Verification items for the finished model (mm, model axes). Coordinates: 2 decimals unless noted, no trailing zeros. Order: outer loops, then holes, each group sorted by start corner. A loop starts at its lowest first (then second) coordinate and runs counter-clockwise, first axis right, second up. Notation, with made-up numbers: M 9,-39 L 50,-39 A24 cw 50,-2 Z; hole C 80.5,7.25 d11. An arc over 180 degrees is marked long. Answer as a JSON object with one key per item and string values. Group by question number.
(1) Cross-section at C-C (y = -2.3). Enter the section's corners in (x, z).
(2) Cross-section at B-B (z = -12). Enter the section's corners in (x, y), plus the area to 3 significant figures.
(3) Cross-section at D-D (x = -10). Enter the section's corners in (y, z), plus the area to 3 significant figures.
(4) Cross-section at A-A (x = 0). Enter the section's corners in (y, z), plus the area to 3 significant figures.
(5) Material ranges on line 1 (Z direction, x = 0, y = 0.95); line 2 (X direction, y = -2.65, z = -1); line 3 (Y direction, x = 2, z = 2.5), recorded low to high.
(6) Gauge pin test, flat ends, axial feed: pin 1 Ø1.5 at (x, y) = (-21.5, -1) entering from +Z; pin 2 Ø2 at (x, y) = (-0.5, -2.5) entering from -Z; pin 3 Ø2.5 at (y, z) = (-2.5, -0.5) entering from -X; pin 4 Ø1.5 at (y, z) = (-1, 0) entering from +X. Record the tip position at first contact, or that the pin passes through.
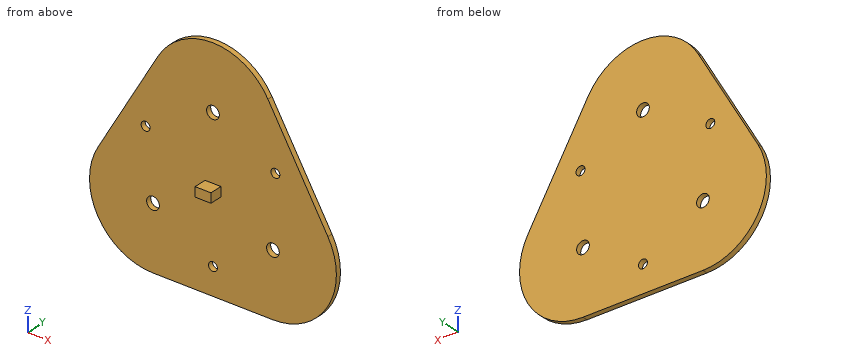
from build123d import *

# Parameters (mm, degrees)
SKETCH1_R           = 2
SKETCH1_R_2         = 1.4
BOSS_EXTRUDE1_DEPTH = 1.65
SKETCH2_W           = 5
SKETCH2_H           = 3
BOSS_EXTRUDE2_DEPTH = 4


with BuildPart() as part:
    # Sketch1 → Boss-Extrude1 (new body)
    with BuildSketch(Plane(origin=(0, 0, 0), x_dir=(1, 0, 0), z_dir=(0, 1, 0))):
        with BuildLine():
            Line((36.224008076, 0.913940814), (17.320508076, -31.827881627))
            ThreePointArc((17.320508076, -31.827881627), (0, -41.827881627), (-17.320508076, -31.827881627))
            Line((-17.320508076, -31.827881627), (-36.224008076, 0.913940814))
            ThreePointArc((-36.224008076, 0.913940814), (-36.224008076, 20.913940814), (-18.9035, 30.913940814))
            Line((-18.9035, 30.913940814), (18.9035, 30.913940814))
            ThreePointArc((18.9035, 30.913940814), (36.224008076, 20.913940814), (36.224008076, 0.913940814))
        make_face()
        with Locations((-18.9035, 10.913940814)):
            Circle(SKETCH1_R, mode=Mode.SUBTRACT)
        with Locations((18.9035, 10.913940814)):
            Circle(SKETCH1_R, mode=Mode.SUBTRACT)
        with Locations((0, -21.827881627)):
            Circle(SKETCH1_R, mode=Mode.SUBTRACT)
        with Locations((-21.238503314, -10.358710199)):
            Circle(SKETCH1_R_2, mode=Mode.SUBTRACT)
        with Locations((19.680254096, -11.3624)):
            Circle(SKETCH1_R_2, mode=Mode.SUBTRACT)
        with Locations((0, 22.3558)):
            Circle(SKETCH1_R_2, mode=Mode.SUBTRACT)
    extrude(amount=BOSS_EXTRUDE1_DEPTH)

    # Sketch2 → Boss-Extrude2 (add)
    with BuildSketch(Plane.XZ):
        Rectangle(SKETCH2_W, SKETCH2_H)
    extrude(amount=BOSS_EXTRUDE2_DEPTH)


solid = part.part
Taken from the geometry:
{
 "1": {"outline": "M -2.5,-1.5 L 2.5,-1.5 L 2.5,1.5 L -2.5,1.5 Z"},
 "2": {"outline": "M -38.87,0 L -20.58,0 L -20.58,1.65 L -38.87,1.65 Z; M -17.22,0 L 17.22,0 L 17.22,1.65 L -17.22,1.65 Z; M 20.58,0 L 38.87,0 L 38.87,1.65 L 20.58,1.65 Z", "area": "117 mm²"},
 "3": {"outline": "M 0,-30.91 L 1.65,-30.91 L 1.65,39.15 L 0,39.15 Z", "area": "116 mm²"},
 "4": {"outline": "M -4,-1.5 L 0,-1.5 L 0,-20.96 L 1.65,-20.96 L 1.65,19.83 L 0,19.83 L 0,1.5 L -4,1.5 Z; M 0,-30.91 L 1.65,-30.91 L 1.65,-23.76 L 0,-23.76 Z; M 0,23.83 L 1.65,23.83 L 1.65,41.83 L 0,41.83 Z", "area": "121 mm²"},
 "5": {"line 1": "z = -30.91 to -23.76, -20.96 to 19.83, 23.83 to 41.83", "line 2": "x = -2.5 to 2.5", "line 3": "y = 0 to 1.65"},
 "6": {"pin 1": "passes through", "pin 2": "stops at z = -1.5", "pin 3": "stops at x = -2.5", "pin 4": "stops at x = 2.5"}
}
